Study the drawing (mm; zero at the part's minimum x, y, z) and answer. A direction names the side the tool comes from. Round coordinates to 2 decimals unless told otherwise and drop trailing zeros. Write each loop counter-clockwise with the first axis right and the second up, starting at its lowest first coordinate (ties: lowest second). Pieces come first, ordered by that corner, then holes.
(1) The mould has two halves that part along Y. Classify the marked faces 1, 2 and 3: +Y half, -Y half, draft (parallel to the pull), parting line (faces both ways), or undercut.
(2) A cutting plane is placed at B-B, the plane y = 21. Give the vertices of the cut face in (x, z).
(3) A cutting plane is placed at A-A, the plane x = 4.5. Give the vertices of the cut face in (y, z), and give its area (3 significant figures).
(4) A cutting plane is placed at D-D, the plane x = 17. Give the vertices of the cut face in (y, z).
(5) A cutting plane is placed at C-C, the plane z = 14. Give the vertices of the cut face in (x, y), and give its area (3 significant figures).
(6) For the marked faces 4 and 5, determine the directions among +Z, -Z, +X, -X, +Y, -Y from which every point of the face is accessible in a straight line to the end or side of a thin tool.
(7) Each of these flat-tipped pins is pushed along its axis until it touches: pin 1 Ø2 at (x, z) = (37.5, 29.5) entering from -Y; pin 2 Ø1.5 at (y, z) = (2, 13.5) entering from +X; pin 3 Ø10 at (x, z) = (32, 22) entering from +Y; pin 4 Ø6 at (x, y) = (25, 15) entering from -Z. Where does it stop, or does it pass through?
(8) Find the intervals of material crossed by probe 1 along X at (y, z) = (16, 9.5); probe 2 along X at (y, z) = (25.25, 9); probe 3 along Y at (x, z) = (40.5, 13.5), in increasing order.
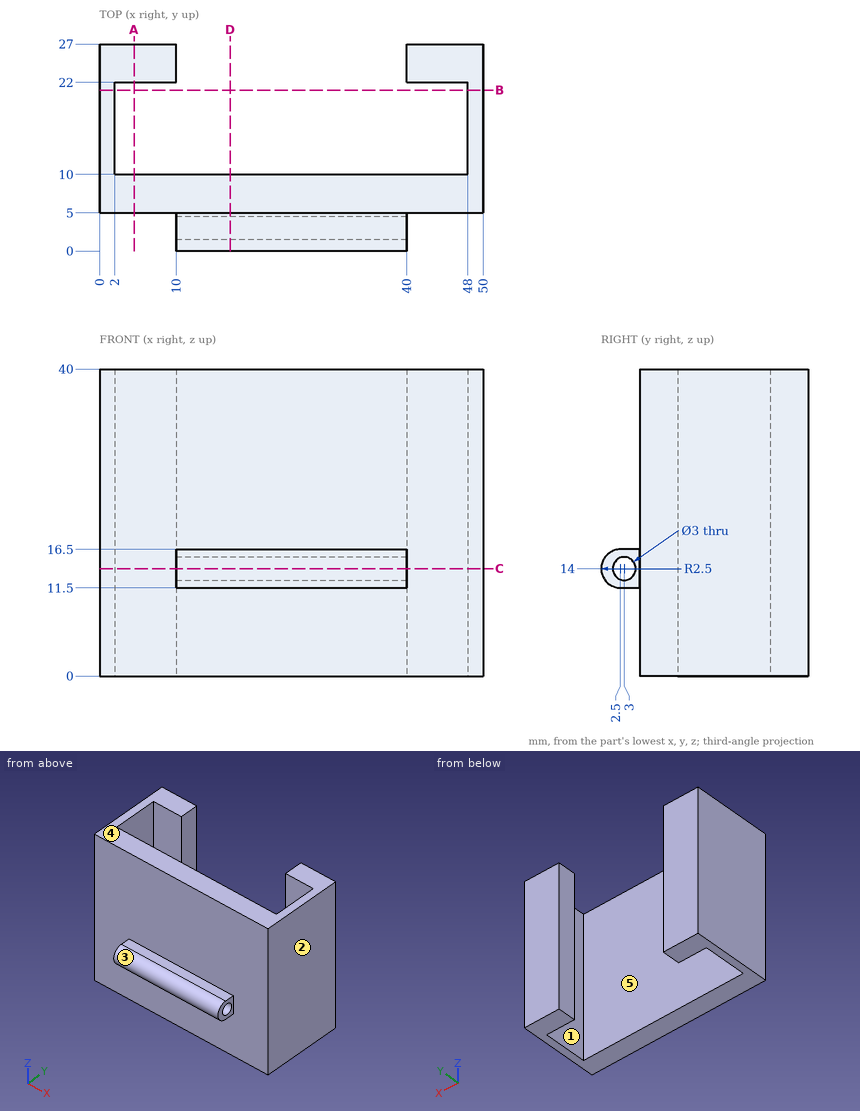
Solutions:
1. face 1: undercut
1. face 2: draft
1. face 3: -Y half
2. outline: (0, 0) - (2, 0) - (2, 40) - (0, 40) - close; (48, 0) - (50, 0) - (50, 40) - (48, 40) - close
3. outline: (5, 0) - (10, 0) - (10, 40) - (5, 40) - close; (22, 0) - (27, 0) - (27, 40) - (22, 40) - close
3. area: 400 mm2
4. outline: (2.5, 11.5) - (5, 11.5) - (5, 0) - (10, 0) - (10, 40) - (5, 40) - (5, 16.5) - (2.5, 16.5) arc R2.5 ccw to start; hole circle Ø3 at (3, 14)
5. outline: (0, 5) - (10, 5) - (10, 4.5) - (40, 4.5) - (40, 5) - (50, 5) - (50, 27) - (40, 27) - (40, 22) - (48, 22) - (48, 10) - (2, 10) - (2, 22) - (10, 22) - (10, 27) - (0, 27) - close; (10, 0) - (40, 0) - (40, 1.5) - (10, 1.5) - close
5. area: 458 mm2
6. face 4: +Z, +X, -X, +Y, -Y
6. face 5: +Z, -Z
7. pin 1: stops at y = 5
7. pin 2: stops at x = 40
7. pin 3: stops at y = 10
7. pin 4: passes through
8. probe 1: x = 0 to 2, 48 to 50
8. probe 2: x = 0 to 10, 40 to 50
8. probe 3: y = 5 to 10, 22 to 27
